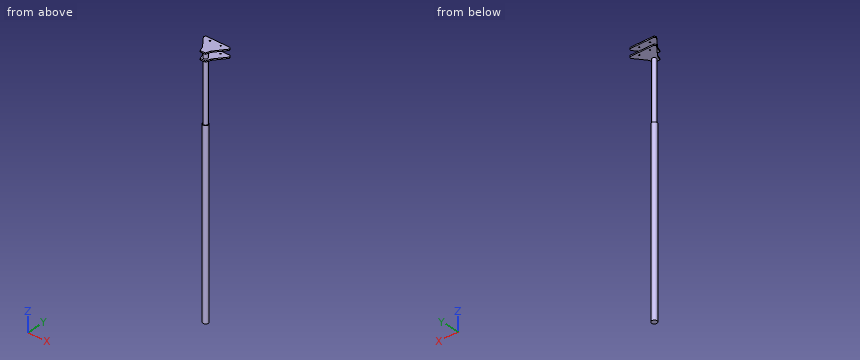
from build123d import *

# Parameters (mm, degrees)
BOSS_EXTRUDE1_START = -380
SKETCH1_R           = 11.3
BOSS_EXTRUDE1_DEPTH = 750
SKETCH2_R           = 8.5
BOSS_EXTRUDE2_DEPTH = 280
BOSS_EXTRUDE3_DEPTH = 5
LPATTERN1_COUNT     = 2
LPATTERN1_PITCH     = 30
SKETCH6_R           = 2.5
CUT_EXTRUDE1_DEPTH  = 150


with BuildPart() as part:
    # Sketch1 → Boss-Extrude1 (new body)
    with BuildSketch(Plane.XY.offset(BOSS_EXTRUDE1_START)):
        Circle(SKETCH1_R)
    extrude(amount=BOSS_EXTRUDE1_DEPTH)

    # Sketch2 → Boss-Extrude2 (add)
    with BuildSketch(Plane.XY.offset(370)):
        Circle(SKETCH2_R)
    extrude(amount=BOSS_EXTRUDE2_DEPTH)

    # Sketch3 → Boss-Extrude3 (add)
    with BuildSketch(Plane.XY.offset(650)):
        Polygon((11.52115326, -14.68790239), (18.072829237, 5.572294102), (55.029019564, 52.840042055), (48.813565956, 60.718856904), (-51.186434044, 60.718856904), (-55.027164938, 52.840905681), (-18.071550308, 5.572707626), (-10.36978253, -14.68790239), (0, -14.68790239), align=None)
    boss_extrude3 = extrude(amount=-BOSS_EXTRUDE3_DEPTH)

    # LPattern1: Boss-Extrude3 ×2
    with Locations(*[(0, 0, -i * LPATTERN1_PITCH) for i in range(1, LPATTERN1_COUNT)]):
        add(boss_extrude3)

    # Sketch6 → Cut-Extrude1 (cut)
    with BuildSketch(Plane.XY.offset(650)):
        with Locations((-23.186517394, 47.937289654)):
            Circle(SKETCH6_R)
        with Locations((20.813649306, 47.937289654)):
            Circle(SKETCH6_R)
    extrude(amount=-CUT_EXTRUDE1_DEPTH, mode=Mode.SUBTRACT)


solid = part.part
The model under review builds one solid part; all positions refer to its coordinate system, in mm. Coordinates: 2 decimals unless noted, no trailing zeros. Write each loop counter-clockwise with the first axis right and the second up, starting at its lowest first coordinate (ties: lowest second). Pieces come first, ordered by that corner, then holes. Notation, with made-up numbers: (54, -33.75) -> (77, -33.75) arc R19 cw to (77, -0.75) -> close; hole circle Ø7 at (17, 75.5). An arc over 180 degrees is marked (long way). Answer in a Markdown table with one row per item.
1. Wall thickness on probe 1 along Z at (x, y) = (0, 10.5); probe 2 along Z at (x, y) = (36, 45); probe 3 along Y at (x, z) = (-1, -11): over which ranges is each line inside the solid? List them lowest first. Write a range as [from, to].
Answers below:
| item | result |
|---|---|
| probe 1 | z = [-380, 370], [615, 620], [645, 650] |
| probe 2 | z = [615, 620], [645, 650] |
| probe 3 | y = [-11.26, 11.26] |
2. We need section D-D, the plane x = 0. State the section outline as (y, z) points, and give its area (3 significant figures).
Answers below:
| item | result |
|---|---|
| outline | (-14.69, 615) -> (-8.5, 615) -> (-8.5, 370) -> (-11.3, 370) -> (-11.3, -380) -> (11.3, -380) -> (11.3, 370) -> (8.5, 370) -> (8.5, 615) -> (60.72, 615) -> (60.72, 620) -> (8.5, 620) -> (8.5, 645) -> (60.72, 645) -> (60.72, 650) -> (-14.69, 650) -> (-14.69, 645) -> (-8.5, 645) -> (-8.5, 620) -> (-14.69, 620) -> close |
| area | 22,300 mm^2 |
3. We need section C-C, the plane z = 287. State the section outline as (x, y) points, and give its area (3 significant figures).
Answers below:
| item | result |
|---|---|
| outline | circle Ø22.6 at (0, 0) |
| area | 401 mm^2 |
4. Clearance check with flat-ended pins moving along their axes: pin 1 Ø1 at (x, z) = (1.5, -256.5) entering from +Y; pin 2 Ø3 at (x, y) = (0.5, 15) entering from -Z; pin 3 Ø2 at (y, z) = (5, 297.5) entering from -X. State where each tip first meets the part, or that it passes through.
Answers below:
| item | result |
|---|---|
| pin 1 | stops at y = 11.26 |
| pin 2 | stops at z = 615 |
| pin 3 | stops at x = -10.57 |
5. We need section B-B, the plane y = 36. State the section outline as (x, z) points, and give its area (3 significant figures).
Answers below:
| item | result |
|---|---|
| outline | (-41.86, 615) -> (41.86, 615) -> (41.86, 620) -> (-41.86, 620) -> close; (-41.86, 645) -> (41.86, 645) -> (41.86, 650) -> (-41.86, 650) -> close |
| area | 837 mm^2 |
6. We need section A-A, the plane x = -40. State the section outline as (y, z) points.
Answers below:
| item | result |
|---|---|
| outline | (33.62, 615) -> (60.72, 615) -> (60.72, 620) -> (33.62, 620) -> close; (33.62, 645) -> (60.72, 645) -> (60.72, 650) -> (33.62, 650) -> close |
